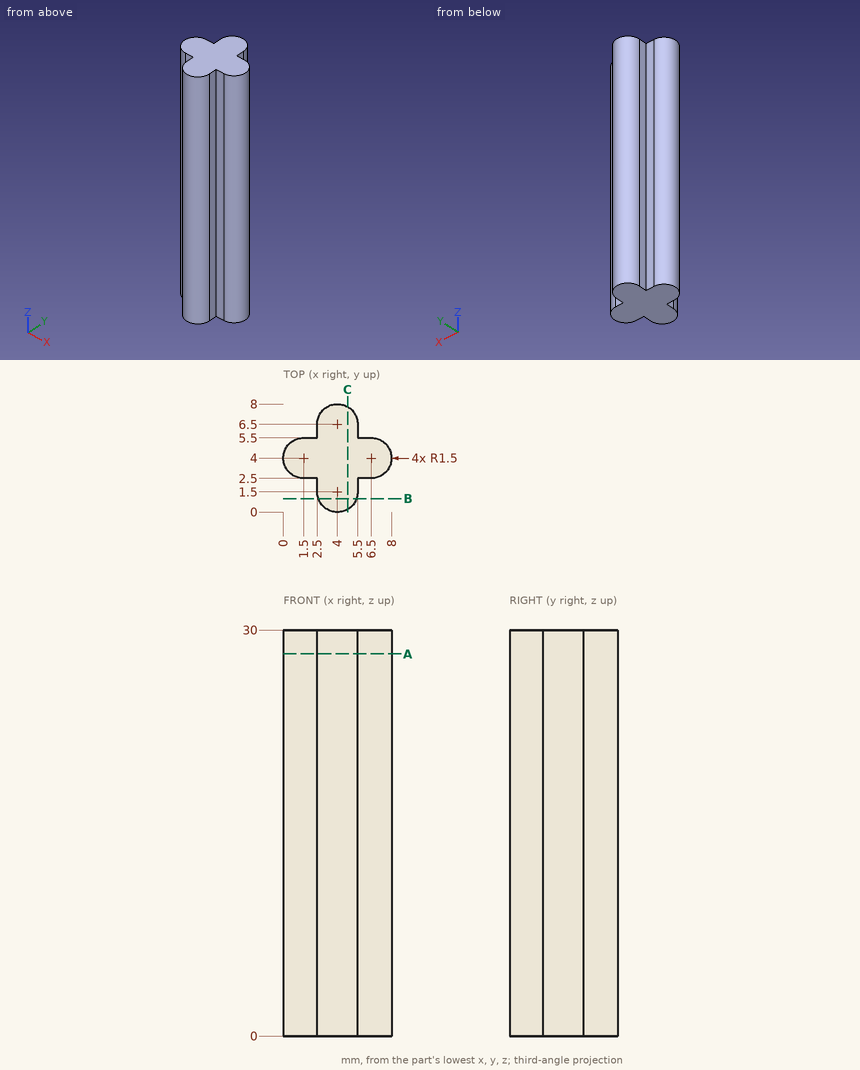
The figure shows three views and two pictorial views of one solid part (mm, origin at its lowest corner). Answer the questions. Give positions to 0.01 mm unless a question says otherwise; leave off trailing zeros. Write each loop counter-clockwise with the first axis right and the second up, starting at its lowest first coordinate (ties: lowest second). Pieces come first, ordered by that corner, then holes.
Q1. The part is cut by section A-A on z = 28.25. Give the vertices of the cut face in (x, y).
Answer:
outline: (1.5, 2.5) - (2.5, 2.5) - (2.5, 1.5) arc R1.5 ccw to (5.5, 1.5) - (5.5, 2.5) - (6.5, 2.5) arc R1.5 ccw to (6.5, 5.5) - (5.5, 5.5) - (5.5, 6.5) arc R1.5 ccw to (2.5, 6.5) - (2.5, 5.5) - (1.5, 5.5) arc R1.5 ccw to start
Q2. Straight lines are drawn through the part: L1, parallel to Y at x = 6.5, z = 24.25; L2, parallel to X at y = 7.75, z = 11.25. For each, find the intervals that lie inside material, in ascending order.
Answer:
L1: y = 2.5 to 5.5
L2: x = 3.17 to 4.83
Q3. The part is cut by section C-C on x = 4.75. Give the vertices of the cut face in (y, z).
Answer:
outline: (0.2, 0) - (7.8, 0) - (7.8, 30) - (0.2, 30) - close
Q4. Given pin 1 (4 mm diameter, centred on x = 6.5, z = 4.5, fed in from -Y); pin 2 (2 mm diameter, centred on x = 2.5, y = 1, fed in from -Z); pin 3 (4 mm diameter, centred on y = 1.5, z = 18, fed in from +X); pin 4 (0.8 mm diameter, centred on x = 6, z = 16.5, fed in from +Y), each flat-ended and moving along its own axis, determine where each tip first touches the part or whether it passes through.
Answer:
pin 1: stops at y = 0.09
pin 2: stops at z = 0
pin 3: stops at x = 7.91
pin 4: stops at y = 5.5
Q5. The part is cut by section B-B on y = 1. Give the vertices of the cut face in (x, z), and give its area (3 significant figures).
Answer:
outline: (2.59, 0) - (5.41, 0) - (5.41, 30) - (2.59, 30) - close
area: 84.9 mm2
